The model under review builds one solid part; all positions refer to its coordinate system, in mm. Coordinates: 2 decimals unless noted, no trailing zeros. Write each loop counter-clockwise with the first axis right and the second up, starting at its lowest first coordinate (ties: lowest second). Pieces come first, ordered by that corner, then holes. Notation, with made-up numbers: (57.5, 48) - (103.5, 48) arc R37 cw to (103.5, 84) - close; hole circle Ø11 at (35, 34). An arc over 180 degrees is marked (long way). Put each result on its own line as item: value.
from build123d import *

# Parameters (mm, degrees)
SKETCH1_W           = 195
SKETCH1_H           = 4
BOSS_EXTRUDE1_DEPTH = 65
CUT_EXTRUDE1_DEPTH  = 10
CUT_EXTRUDE2_DEPTH  = 10


with BuildPart() as part:
    # Sketch1 → Boss-Extrude1 (new body)
    with BuildSketch(Plane(origin=(0, 0, 0), x_dir=(1, 0, 0), z_dir=(0, 1, 0))):
        Rectangle(SKETCH1_W, SKETCH1_H)
    extrude(amount=-BOSS_EXTRUDE1_DEPTH)

    # Sketch2 → Cut-Extrude1 (cut)
    with BuildSketch(Plane.XY.offset(2)):
        Polygon((-97.5, 0), (97.5, -20), (97.5, 0), align=None)
    extrude(amount=-CUT_EXTRUDE1_DEPTH, mode=Mode.SUBTRACT)

    # Sketch3 → Cut-Extrude2 (cut)
    with BuildSketch(Plane.XY.offset(2)):
        with BuildLine():
            Line((-97.5, -20), (-97.5, -65))
            Line((-97.5, -65), (-52.5, -65))
            ThreePointArc((-52.5, -65), (-84.319805153, -51.819805153), (-97.5, -20))
        make_face()
    extrude(amount=-CUT_EXTRUDE2_DEPTH, mode=Mode.SUBTRACT)


solid = part.part
1. For pin 1 Ø1.5 at (x, z) = (-43, -0.5) entering from +Y; pin 2 Ø2 at (x, z) = (36.5, 0.5) entering from +Y, all flat-tipped, find the tip position at first contact; note any pin that passes through.
Determined:
pin 1: stops at y = -5.51
pin 2: stops at y = -13.64
2. Consider section A-A on z = 0.7. State the section outline as (x, y) points, plus the area to 3 significant figures.
Determined:
outline: (-97.5, -20) arc R45 ccw to (-52.5, -65) - (97.5, -65) - (97.5, -20) - (-97.5, 0) - close
area: 10,300 mm^2
3. Consider section C-C on x = -78. State the section outline as (y, z) points.
Determined:
outline: (-57.08, -2) - (-2, -2) - (-2, 2) - (-57.08, 2) - close
4. To check wall thickness, follow probe 1 along Y at (x, z) = (75.5, 1.3); probe 2 along X at (y, z) = (-40, -1.05); probe 3 along X at (y, z) = (-23, 0.15). State the ranges of each line that lie inside material, in increasing order.
Determined:
probe 1: y = -65 to -17.74
probe 2: x = -92.81 to 97.5
probe 3: x = -97.4 to 97.5
5. Consider section B-B on y = -51. State the section outline as (x, z) points.
Determined:
outline: (-85.12, -2) - (97.5, -2) - (97.5, 2) - (-85.12, 2) - close
